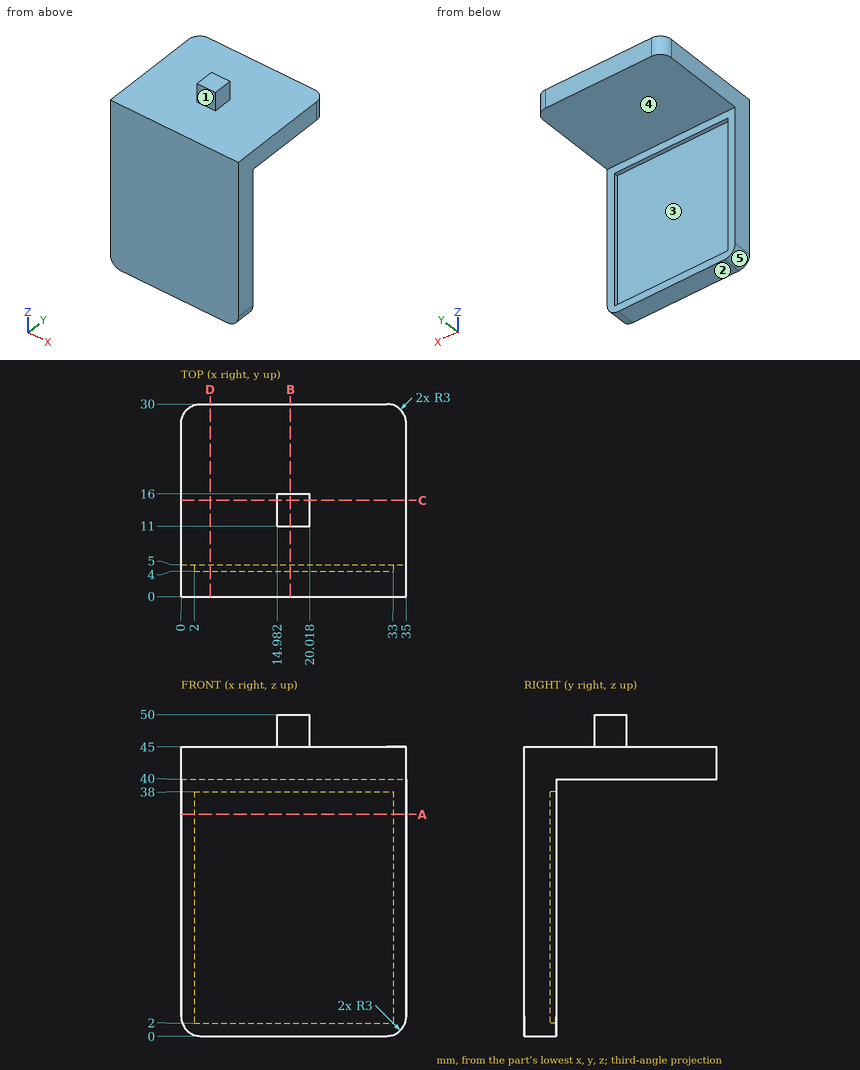
Drawing for the job (mm, zero at the part's lowest x, y, z). A direction names the side the tool comes from. Give positions to 0.01 mm unless a question says otherwise; leave off trailing zeros. Order: outer loops, then holes, each group sorted by start corner. A loop starts at its lowest first (then second) coordinate and runs counter-clockwise, first axis right, second up. Notation, with made-up numbers: M 71.5,50.5 L 121.5,50.5 A30 cw 121.5,74.5 Z; hole C 82,62.5 d4. An arc over 180 degrees is marked long. Put each result on its own line as item: value.
Item 1: Slice it at C-C, the plane y = 15. Write the cut outline in (x, z), plus the area to 3 significant figures.
From the geometry:
outline: M 0,40 L 35,40 L 35,45 L 20.02,45 L 20.02,50 L 14.98,50 L 14.98,45 L 0,45 Z
area: 200 mm2
Item 2: Flat gauge pins, fed straight in: pin 1 Ø8 at (x, z) = (24, 18.5) entering from +Y; pin 2 Ø1.5 at (x, z) = (17.5, 48) entering from +Y; pin 3 Ø0.8 at (x, y) = (22, 4.5) entering from +Z. Where does each tip first touch, or does it go through?
From the geometry:
pin 1: stops at y = 4
pin 2: stops at y = 16
pin 3: stops at z = 45
Item 3: Probe line 1 (Z direction, x = 31, y = 4.75); line 2 (Y direction, x = 22.5, z = 39); line 3 (Y direction, x = 10, z = 20). List the from-to ranges inside material, lowest first. Write a range as [from, to].
From the geometry:
line 1: z = [0, 2], [38, 45]
line 2: y = [0, 5]
line 3: y = [0, 4]
Item 4: Two-plate mould, pull along X, no slides. Class the marked faces 3, 4 and 5: +X half, -X half, draft (parallel to the pull), parting line (faces both ways), or undercut.
From the geometry:
face 3: undercut
face 4: draft
face 5: -X half
Item 5: Slice it at B-B, the plane x = 17. Write the cut outline in (y, z).
From the geometry:
outline: M 0,0 L 5,0 L 5,2 L 4,2 L 4,38 L 5,38 L 5,40 L 30,40 L 30,45 L 16,45 L 16,50 L 11,50 L 11,45 L 0,45 Z
Item 6: Slice it at D-D, the plane x = 4.5. Write the cut outline in (y, z).
From the geometry:
outline: M 0,0 L 5,0 L 5,2 L 4,2 L 4,38 L 5,38 L 5,40 L 30,40 L 30,45 L 0,45 Z
Item 7: 3-axis set-ups, long thin cutter, end or side, ignore diameter. For the marked faces 1 and 2: which of +Z, -Z, +X, -X, +Y, -Y reach the whole face in a straight line?
From the geometry:
face 1: +Z, +X, -X, -Y
face 2: -Z, +X, -X, +Y, -Y
Item 8: Slice it at A-A, the plane z = 34.5. Write the cut outline in (x, y), plus the area to 3 significant figures.
From the geometry:
outline: M 0,0 L 35,0 L 35,5 L 33,5 L 33,4 L 2,4 L 2,5 L 0,5 Z
area: 144 mm2
